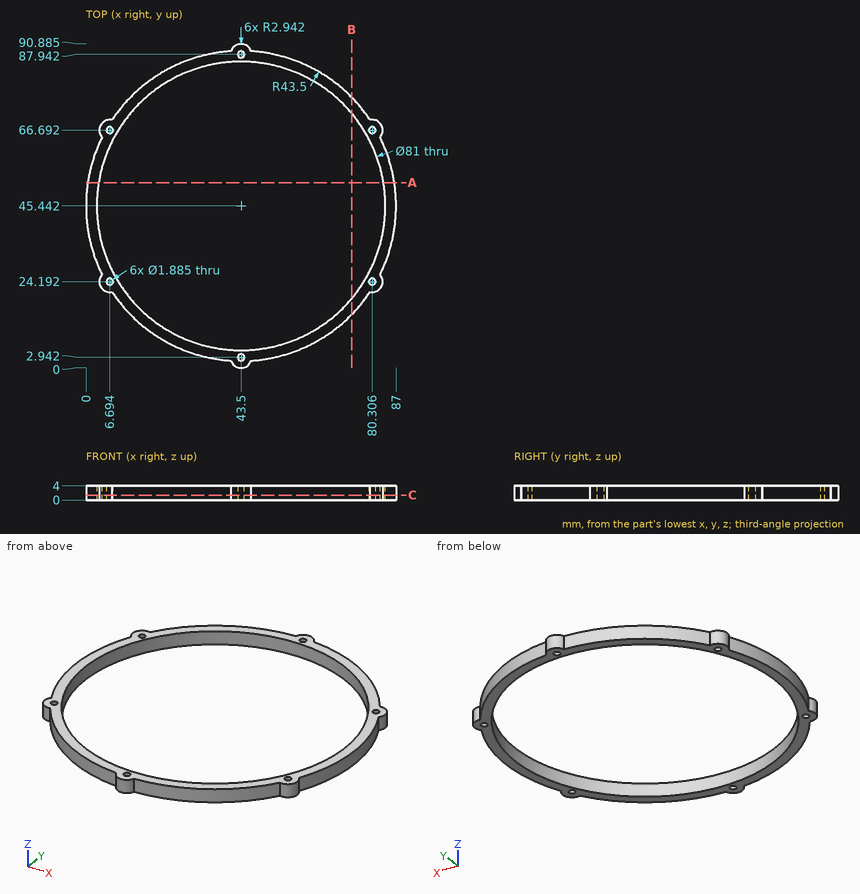
Job drawing, mm, ordinate dimensions from the low corner. One solid piece. Coordinates: 2 decimals unless noted, no trailing zeros. Write each loop counter-clockwise with the first axis right and the second up, starting at its lowest first coordinate (ties: lowest second). Pieces come first, ordered by that corner, then holes. Notation, with made-up numbers: (-2.75, -38.5) -> (53.25, -38.5) arc R32 cw to (53.25, -9.5) -> close; hole circle Ø2 at (87.25, 15). An arc over 180 degrees is marked (long way). Use CSV: the item, a comma, the result in double quotes. Start each with the question number.
Item 1: Band-saw the part on C-C, the plane z = 1.4. Write the cut outline in (x, y) (1 decimal).
Item 2: Drop flat-ended pins along their axis: P1, Ø1.5, axis at y = 33.5, z = 3, coming from the +X side (1 decimal); P2, Ø2, axis at y = 64, z = 1.5, coming from the +X side; P3, Ø1.1, axis at x = 6.69, y = 66.69, coming from the +Z side; P4, Ø1.5, axis at y = 9.5, z = 3.5, coming from the +X side. Give the stop position or say it passes through.
Item 3: Wall check: probe 1 along Y at (x, z) = (43.5, 2.2) (1 decimal); probe 2 along Y at (x, z) = (45, 3) (1 decimal); probe 3 along X at (y, z) = (36.5, 3). Give the ranges that are in metal, low to high.
Item 4: Band-saw the part on B-B, the plane x = 74.5. Write the cut outline in (y, z) (1 decimal).
Item 5: Band-saw the part on A-A, the plane y = 52. Write the cut outline in (x, z) (1 decimal), plus the area to 3 significant figures.
Response values:
1,outline,"(4.5, 26.2) arc R2.9 ccw to (7.3, 21.3) arc R43.5 ccw to (40.7, 2) arc R2.9 ccw to (46.3, 2) arc R43.5 ccw to (79.7, 21.3) arc R2.9 ccw to (82.5, 26.2) arc R43.5 ccw to (82.5, 64.7) arc R2.9 ccw to (79.7, 69.6) arc R43.5 ccw to (46.3, 88.9) arc R2.9 ccw to (40.7, 88.9) arc R43.5 ccw to (7.3, 69.6) arc R2.9 ccw to (4.5, 64.7) arc R43.5 ccw to start; hole circle Ø81 at (43.5, 45.4); hole circle Ø1.9 at (6.7, 24.2); hole circle Ø1.9 at (6.7, 66.7); hole circle Ø1.9 at (43.5, 2.9); hole circle Ø1.9 at (43.5, 87.9); hole circle Ø1.9 at (80.3, 24.2); hole circle Ø1.9 at (80.3, 66.7)"
2,P1,"stops at x = 85.5"
2,P2,"stops at x = 83.3"
2,P3,"passes through"
2,P4,"stops at x = 69.07"
3,probe 1,"y = 0 to 2, 3.9 to 4.9, 85.9 to 87, 88.9 to 90.9"
3,probe 2,"y = 0.4 to 5, 85.9 to 90.5"
3,probe 3,"x = 0.93 to 4, 83 to 86.07"
4,outline,"(14.9, 0) -> (19.4, 0) -> (19.4, 4) -> (14.9, 4) -> close; (71.5, 0) -> (76, 0) -> (76, 4) -> (71.5, 4) -> close"
5,outline,"(0.5, 0) -> (3.5, 0) -> (3.5, 4) -> (0.5, 4) -> close; (83.5, 0) -> (86.5, 0) -> (86.5, 4) -> (83.5, 4) -> close"
5,area,"24.3 mm2"
